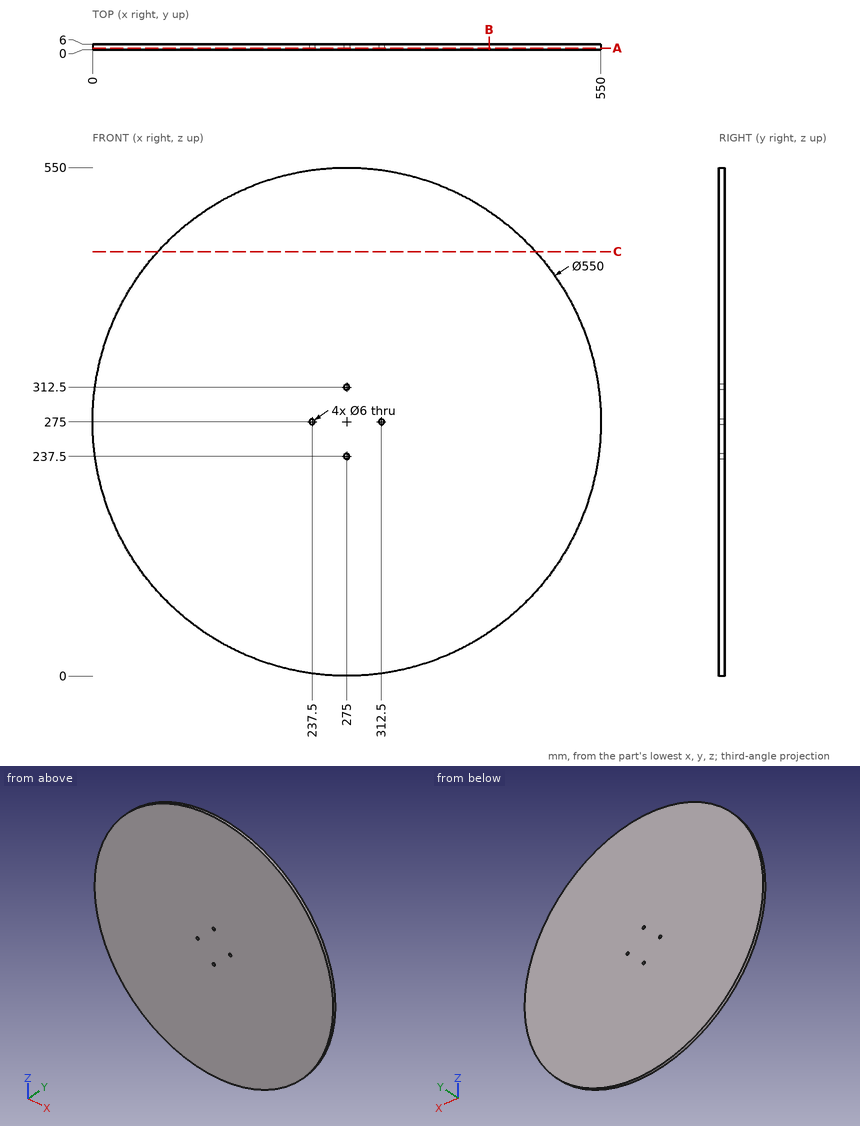
For this review, use the dimensioned drawing (mm, ordinates from the lowest corner) and the shaded views. Round coordinates to 2 decimals unless told otherwise and drop trailing zeros. Order: outer loops, then holes, each group sorted by start corner. A loop starts at its lowest first (then second) coordinate and runs counter-clockwise, first axis right, second up. Notation, with made-up numbers: M 81.5,-37.75 L 87.5,-37.75 A18 cw 87.5,-10.75 Z; hole C 41,39.5 d9. An arc over 180 degrees is marked long. Use a Markdown table: item, result.
1) Consider section C-C (z = 459). Write out the cut boundary in (x, y), then the cut area to 3 significant figures.
Report:
| item | result |
|---|---|
| outline | M 70.63,0 L 479.37,0 L 479.37,6 L 70.63,6 Z |
| area | 2,450 mm^2 |
2) Consider section B-B (x = 429). Write out the cut boundary in (y, z).
Report:
| item | result |
|---|---|
| outline | M 0,47.16 L 6,47.16 L 6,502.84 L 0,502.84 Z |
3) Wall thickness on line 1 along X through (y, z) = (4, 275); line 2 along X through (y, z) = (3.6, 237.5); line 3 along X through (y, z) = (0.8, 111): over which ranges is each line inside the solid? List them lowest first. Write a range as [from, to].
Report:
| item | result |
|---|---|
| line 1 | [0, 234.5], [240.5, 309.5], [315.5, 550] |
| line 2 | [2.57, 272], [278, 547.43] |
| line 3 | [54.25, 495.75] |
4) Consider section A-A (y = 1.4). Write out the cut boundary in (x, z).
Report:
| item | result |
|---|---|
| outline | C 275,275 d550; hole C 237.5,275 d6; hole C 275,237.5 d6; hole C 275,312.5 d6; hole C 312.5,275 d6 |
5) Insertion check: pin 1 (2 mm diameter, centred on x = 358, y = 2, fed in from -Z); pin 2 (5.5 mm diameter, centred on x = 275, z = 237.5, fed in from -Y). Each pin has a flat end and moves straight along its axis. Give the tip position at first contact, or say it passes through.
Report:
| item | result |
|---|---|
| pin 1 | z = 12.51 |
| pin 2 | through |
